Part model, mm, in its own coordinate system. Face numbers are marked on the shaded views. A direction names the side the tool comes from. Round coordinates to 2 decimals unless told otherwise and drop trailing zeros. Write each loop counter-clockwise with the first axis right and the second up, starting at its lowest first coordinate (ties: lowest second). Pieces come first, ordered by that corner, then holes. Notation, with made-up numbers: (40.25, -12) -> (72.25, -12) arc R21 cw to (72.25, 11) -> close; hole circle Ø2 at (-20.5, 58). An arc over 180 degrees is marked (long way). Return JSON: item names as keys, results as strings. Group by question number.
(1) Saw through at A-A (z = -8). List the corners of the cut face in (x, y).
(2) Saw through at C-C (y = 38). List the corners of the cut face in (x, z), plus the area to 3 significant figures.
(3) Tool access for the marked faces 5 and 6: list every direction of +Z, -Z, +X, -X, +Y, -Y with a clear straight run to the whole face (end or side of a thin tool).
(4) Mould opens along Z. For the marked faces 1, 2, 3 and 4 say: +Z half, -Z half, draft (parallel to the pull), parting line (faces both ways), or undercut.
(5) Saw through at D-D (z = -6.25). List the corners of the cut face in (x, y).
(6) Drill centre lines: L1, parallel to Y at x = 3.05, z = -8.5; L2, parallel to Z at x = 3.4, y = 39.5; L3, parallel to Z at x = 2.7, y = 30.5. Where is each one in solid material? Low to high. Write a range as from..to.
(7) Saw through at B-B (x = 3.1). List the corners of the cut face in (y, z), plus the area to 3 significant figures.
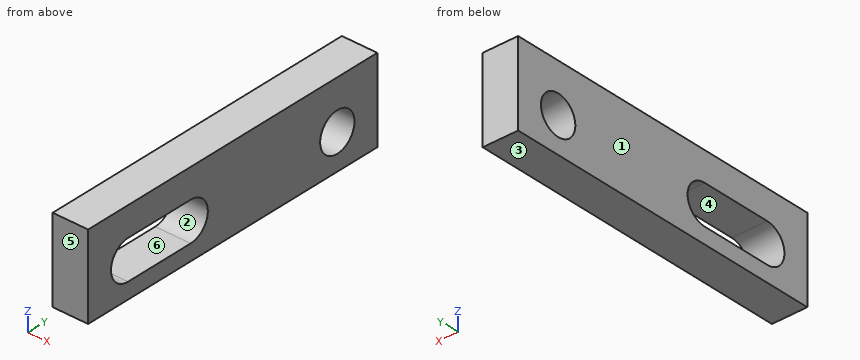
Solid Edge part; units mm, degrees
sketch "Sketch1" plane through (0, 0, 0) normal (1, 0, 0) x (0, 1, 0)
  line L0 (63.3741, -12) -> (63.3741, -2.5)
  line L1 (63.3741, -2.5) -> (26.3156, -2.5)
  line L2 (26.3156, -2.5) -> (26.3156, -12)
  line L3 (26.3156, -12) -> (63.3741, -12)
  line L4 (39.4564, -10.2) -> (31.4456, -10.2)
  arc A0 (39.4564, -5.8) -> (39.4564, -10.2) centre (39.4564, -8) cw
  line L5 (31.4456, -5.8) -> (39.4564, -5.8)
  arc A1 (31.4456, -10.2) -> (31.4456, -5.8) centre (31.4456, -8) cw
  circle A2 centre (58.2478, -8) radius 2.2
extrude "Protrusion1" add sketch "Sketch1" along normal blind 4
Computed values:
{
 "1": {"outline": "(0, 26.32) -> (4, 26.32) -> (4, 29.25) -> (0, 29.25) -> close; (0, 41.66) -> (4, 41.66) -> (4, 56.05) -> (0, 56.05) -> close; (0, 60.45) -> (4, 60.45) -> (4, 63.37) -> (0, 63.37) -> close"},
 "2": {"outline": "(0, -12) -> (4, -12) -> (4, -10.2) -> (0, -10.2) -> close; (0, -5.8) -> (4, -5.8) -> (4, -2.5) -> (0, -2.5) -> close", "area": "20.4 mm2"},
 "3": {"face 5": "+Z, -Z, +X, -X, -Y", "face 6": "+X, -X"},
 "4": {"face 1": "draft", "face 2": "undercut", "face 3": "-Z half", "face 4": "undercut"},
 "5": {"outline": "(0, 26.32) -> (4, 26.32) -> (4, 30.11) -> (0, 30.11) -> close; (0, 40.79) -> (4, 40.79) -> (4, 56.91) -> (0, 56.91) -> close; (0, 59.58) -> (4, 59.58) -> (4, 63.37) -> (0, 63.37) -> close"},
 "6": {"L1": "26.32..29.3, 41.6..56.11, 60.39..63.37", "L2": "-12..-10.2, -5.8..-2.5", "L3": "-12..-9.99, -6.01..-2.5"},
 "7": {"outline": "(26.32, -12) -> (63.37, -12) -> (63.37, -2.5) -> (26.32, -2.5) -> close; hole (31.45, -10.2) -> (39.46, -10.2) arc R2.2 ccw to (39.46, -5.8) -> (31.45, -5.8) arc R2.2 ccw to start; hole circle Ø4.4 at (58.25, -8)", "area": "286 mm2"}
}
